Build history of the part. All positions in model axes, mm. Face numbers are marked on the shaded views. A direction names the side the tool comes from. Coordinates: 2 decimals unless noted, no trailing zeros. Loops run counter-clockwise (first coordinate to the right, second up) from the corner with the lowest first, then second, coordinate; pieces in that order, holes last. Notation, with made-up numbers: (-36.75, -10.5) - (-20.75, -10.5) arc R11 ccw to (-20.75, -1.5) - close; hole circle Ø1 at (43.5, -40). An arc over 180 degrees is marked (long way). One line per item, written item: value.
```python
from build123d import *

# Parameters (mm, degrees)
BOSS_EXTRUDE1_DEPTH = 50.8
SKETCH2_R           = 2.6035
CUT_EXTRUDE1_DEPTH  = 5.08
FILLET1_R           = 5.08


with BuildPart() as part:
    # Sketch1 → Boss-Extrude1 (new body)
    with BuildSketch(Plane.XY):
        Polygon((12.7, 54.4576), (12.7, 70.3326), (53.721, 70.3326), (53.721, 54.4576), (59.1185, 54.4576), (59.1185, 52.6288), (53.721, 52.6288), (53.721, 36.7538), (59.1185, 36.7538), (59.1185, 34.925), (53.721, 34.925), (53.721, 0), (72.771, 0), (72.771, 15.572598677), (68.2498, 15.572598677), (68.2498, 11.0236), (66.421, 11.0236), (66.421, 15.572598677), (62.23, 15.572598677), (62.23, 58.752598677), (66.421, 58.752598677), (66.421, 62.7126), (68.2498, 62.7126), (68.2498, 58.752598677), (72.771, 58.752598677), (72.771, 74.1426), (66.421, 74.1426), (66.421, 81.7626), (54.8005, 81.7626), (54.8005, 78.5876), (61.1505, 78.5876), (61.1505, 74.1426), (5.2705, 74.1426), (5.2705, 78.5876), (11.6205, 78.5876), (11.6205, 81.7626), (0, 81.7626), (0, 0), (12.7, 0), (12.7, 34.925), (7.3025, 34.925), (7.3025, 36.7538), (12.7, 36.7538), (12.7, 52.6288), (7.3025, 52.6288), (7.3025, 54.4576), align=None)
    extrude(amount=BOSS_EXTRUDE1_DEPTH)

    # Sketch2 → Cut-Extrude1 (cut)
    with BuildSketch(Plane.XZ):
        with Locations((6.35, 44.45)):
            Circle(SKETCH2_R)
        with Locations((66.421, 6.35)):
            Circle(SKETCH2_R)
    extrude(amount=-CUT_EXTRUDE1_DEPTH, mode=Mode.SUBTRACT)

    # Fillet1
    fillet1_edges = [part.edges().sort_by_distance(p)[0] for p in [
        (53.721, 70.3326, 25.4),
        (12.7, 70.3326, 25.4),
        (0, 81.7626, 25.4),
        (66.421, 81.7626, 25.4),
        (72.771, 74.1426, 25.4),
    ]]
    fillet(fillet1_edges, radius=FILLET1_R)


solid = part.part
```
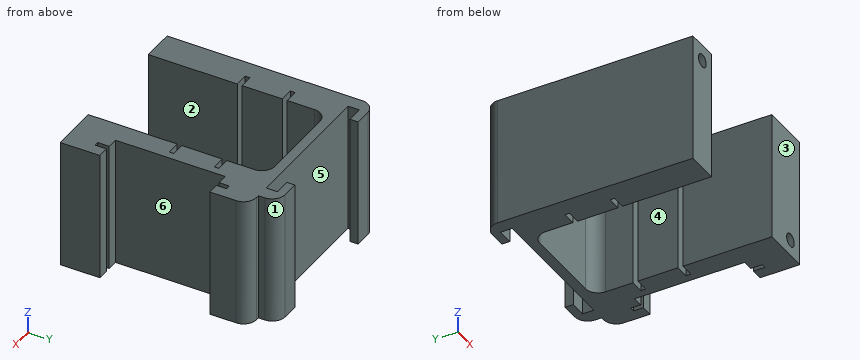
Item 1: Pull direction X, two halves, no side cores. Call the marked faces 1, 2 and 3: released by +X, released by -X, zero draft, split by the parting line, or undercut.
Check result:
face 1: released by +X
face 2: undercut
face 3: zero draft
Item 2: Cut at A-A, the plane y = 29. Write the cut outline in (x, z), then the cut area to 3 significant figures.
Check result:
outline: (0, 0) - (12.7, 0) - (12.7, 50.8) - (0, 50.8) - close; (53.72, 0) - (62.23, 0) - (62.23, 50.8) - (53.72, 50.8) - close
area: 1,080 mm^2
Item 3: Probe probe 1 along Y at (x, z) = (10, 36) (3 decimals); probe 2 along X at (y, z) = (55, 10); probe 3 along Z at (x, y) = (6, 2). List the from-to ranges inside material, lowest first. Write a range as from..to.
Check result:
probe 1: y = 0..34.925, 36.754..52.629, 54.458..74.143, 78.588..81.763
probe 2: x = 0..12.7, 53.72..62.23
probe 3: z = 0..41.87, 47.03..50.8
Item 4: Tool access for the marked faces 4, 5 and 6: list every direction of +Z, -Z, +X, -X, +Y, -Y with a clear straight run to the whole face (end or side of a thin tool).
Check result:
face 4: +Z, -Z, -Y
face 5: +Z, -Z
face 6: +Z, -Z, +X
Item 5: Drop flat-ended pins along their axis: P1, Ø4, axis at x = 51.5, z = 31.5, coming from the +Y side; P2, Ø2, axis at x = 54, z = 30.5, coming from the +Y side; P3, Ø4.5, axis at x = 6.35, z = 44.45, coming from the -Y side; P4, Ø4, axis at y = 71.5, z = 44, coming from the +X side. Give the stop position or say it passes through.
Check result:
P1: stops at y = 74.14
P2: stops at y = 81.76
P3: stops at y = 5.08
P4: stops at x = 72.75
